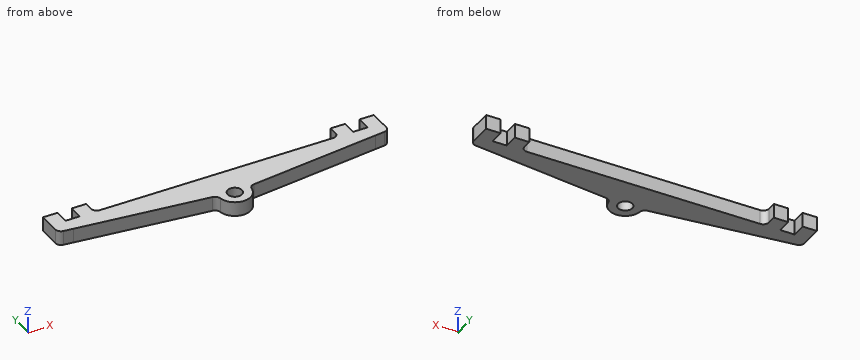
from build123d import *

# Parameters (mm, degrees)
SKETCH1_R      = 3.175
EXTRUDE1_DEPTH = 6.35


with BuildPart() as part:
    # Sketch1 → Extrude1 (new body)
    with BuildSketch(Plane.XY):
        with BuildLine():
            Line((-66.675, 8.128), (-9.141527829, 1.269026149))
            ThreePointArc((-9.141527829, 1.269026149), (-7.658129481, 0.554828765), (-6.924287371, -0.91895016))
            ThreePointArc((-6.924287371, -0.91895016), (0, -6.985), (6.924287371, -0.91895016))
            ThreePointArc((6.924287371, -0.91895016), (7.658129481, 0.554828765), (9.141527829, 1.269026149))
            Line((9.141527829, 1.269026149), (66.675, 8.128))
            Line((66.675, 8.128), (70.785682223, 8.618063624))
            ThreePointArc((70.785682223, 8.618063624), (72.384385802, 9.453807003), (73.025, 11.140203628))
            Line((73.025, 11.140203628), (73.025, 20.828))
            Line((73.025, 20.828), (66.675, 20.828))
            Line((66.675, 20.828), (66.675, 14.478))
            Line((66.675, 14.478), (60.325, 14.478))
            Line((60.325, 14.478), (60.325, 20.828))
            Line((60.325, 20.828), (53.975, 20.828))
            Line((53.975, 20.828), (53.975, 17.018))
            ThreePointArc((53.975, 17.018), (53.231051224, 15.221948776), (51.435, 14.478))
            Line((51.435, 14.478), (-51.435, 14.478))
            ThreePointArc((-51.435, 14.478), (-53.231051224, 15.221948776), (-53.975, 17.018))
            Line((-53.975, 17.018), (-53.975, 20.828))
            Line((-53.975, 20.828), (-60.325, 20.828))
            Line((-60.325, 20.828), (-60.325, 14.478))
            Line((-60.325, 14.478), (-66.675, 14.478))
            Line((-66.675, 14.478), (-66.675, 20.828))
            Line((-66.675, 20.828), (-73.025, 20.828))
            Line((-73.025, 20.828), (-73.025, 11.140203628))
            ThreePointArc((-73.025, 11.140203628), (-72.384385802, 9.453807003), (-70.785682223, 8.618063624))
            Line((-70.785682223, 8.618063624), (-66.675, 8.128))
        make_face()
        Circle(SKETCH1_R, mode=Mode.SUBTRACT)
    extrude(amount=EXTRUDE1_DEPTH)


solid = part.part
Build history of the part. All positions in model axes, mm. Coordinates: 2 decimals unless noted, no trailing zeros. Write each loop counter-clockwise with the first axis right and the second up, starting at its lowest first coordinate (ties: lowest second). Pieces come first, ordered by that corner, then holes.
(1) Cut at B-B on y = 18.5. List the corners of the cut face in (x, z) (3 decimals).
(2) Cut at D-D on y = 6. List the corners of the cut face in (x, z).
(3) Cut at C-C on z = 5. List the corners of the cut face in (x, y) (3 decimals).
(4) Drill centre lines: line 1 (X direction, y = 18.75, z = 5) (3 decimals); line 2 (Y direction, x = 0, z = 1.5) (3 decimals); line 3 (Y direction, x = 47.5, z = 5). Where is each one in solid material? Low to high.
(5) Pin check, flat tips, straight feed: pin 1 Ø3 at (x, z) = (64, 4.5) entering from +Y; pin 2 Ø2 at (y, z) = (-4, 3) entering from -X; pin 3 Ø3 at (y, z) = (-2, 1) entering from -X. Stop position of each tip, or through.
(6) Cut at A-A on x = 0. List the corners of the cut face in (y, z) (3 decimals).
Working result:
1. outline: (-73.025, 0) - (-66.675, 0) - (-66.675, 6.35) - (-73.025, 6.35) - close; (-60.325, 0) - (-53.975, 0) - (-53.975, 6.35) - (-60.325, 6.35) - close; (53.975, 0) - (60.325, 0) - (60.325, 6.35) - (53.975, 6.35) - close; (66.675, 0) - (73.025, 0) - (73.025, 6.35) - (66.675, 6.35) - close
2. outline: (-48.83, 0) - (48.83, 0) - (48.83, 6.35) - (-48.83, 6.35) - close
3. outline: (-73.025, 11.14) arc R2.54 ccw to (-70.786, 8.618) - (-9.142, 1.269) arc R2.54 cw to (-6.924, -0.919) arc R6.985 ccw to (6.924, -0.919) arc R2.54 cw to (9.142, 1.269) - (70.786, 8.618) arc R2.54 ccw to (73.025, 11.14) - (73.025, 20.828) - (66.675, 20.828) - (66.675, 14.478) - (60.325, 14.478) - (60.325, 20.828) - (53.975, 20.828) - (53.975, 17.018) arc R2.54 cw to (51.435, 14.478) - (-51.435, 14.478) arc R2.54 cw to (-53.975, 17.018) - (-53.975, 20.828) - (-60.325, 20.828) - (-60.325, 14.478) - (-66.675, 14.478) - (-66.675, 20.828) - (-73.025, 20.828) - close; hole circle Ø6.35 at (0, 0)
4. line 1: x = -73.025 to -66.675, -60.325 to -53.975, 53.975 to 60.325, 66.675 to 73.025
4. line 2: y = -6.985 to -3.175, 3.175 to 14.478
4. line 3: y = 5.84 to 14.48
5. pin 1: stops at y = 14.48
5. pin 2: stops at x = -6.31
5. pin 3: stops at x = -7.02
6. outline: (-6.985, 0) - (-3.175, 0) - (-3.175, 6.35) - (-6.985, 6.35) - close; (3.175, 0) - (14.478, 0) - (14.478, 6.35) - (3.175, 6.35) - close
